Model file for the job. Use its own axes, mm. Coordinates: 2 decimals unless noted, no trailing zeros. Order: outer loops, then holes, each group sorted by start corner. A loop starts at its lowest first (then second) coordinate and runs counter-clockwise, first axis right, second up. Notation, with made-up numbers: (66.5, 88) -> (108.5, 88) arc R13 ccw to (108.5, 92) -> close; hole circle Ø11 at (84.5, 35.25). An arc over 180 degrees is marked (long way). Return JSON: item names as keys, results as strings. Group by question number.
1) Probe line 1 (Z direction, x = 9, y = -0.3); line 2 (Z direction, x = 30.5, y = -0.4); line 3 (X direction, y = -0.35, z = -22). List the from-to ranges inside material, lowest first.
2) Cut at D-D (x = 19). Write the cut outline in (y, z).
3) Cut at B-B (y = -0.05). Write the cut outline in (x, z).
4) Cut at C-C (z = -50). Write the cut outline in (x, y).
5) Flat gauge pins, fed straight in: pin 1 (3.5 mm diameter, centred on x = 9, z = 40, fed in from -Y); pin 2 (0.5 mm diameter, centred on x = 29.5, y = 0, fed in from +Z). Where does each tip first touch, or does it go through?
6) Cut at A-A (z = 77). Write the cut outline in (x, y).
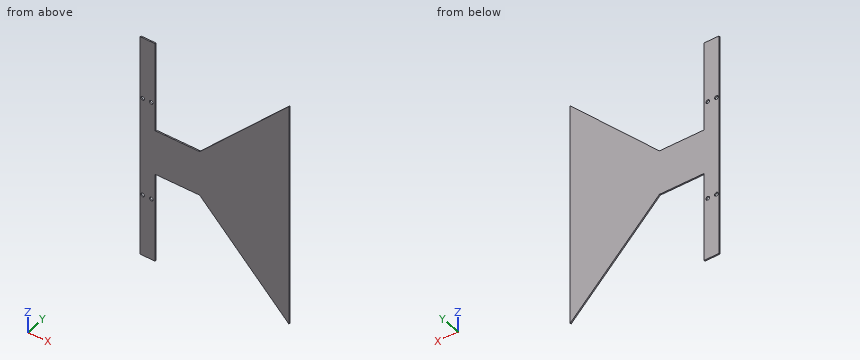
from build123d import *

# Parameters (mm, degrees)
F0_R     = 1.5
F0_W     = 36
F0_H     = 36
F1_DEPTH = 0.5


with BuildPart() as f1:
    # F0 (on Front) → F1 (new body, symmetric)
    with BuildSketch(Plane.XZ):
        Polygon((12, 90), (0, 90), (0, -90), (12, -90), (12, -18), (12, 18), align=None)
        with Locations((2, -40)):
            Circle(F0_R, mode=Mode.SUBTRACT)
        with Locations((9, -40)):
            Circle(F0_R, mode=Mode.SUBTRACT)
        with Locations((2, 40)):
            Circle(F0_R, mode=Mode.SUBTRACT)
        with Locations((9, 40)):
            Circle(F0_R, mode=Mode.SUBTRACT)
        with Locations((30, 0)):
            Rectangle(F0_W, F0_H)
        Polygon((120, 90), (48, 18), (48, -18), (120, -90), align=None)
    extrude(amount=F1_DEPTH, both=True)


solid = f1.part
Answers below:
{
 "1": {"line 1": "z = -90 to -41.5, -38.5 to 38.5, 41.5 to 90", "line 2": "z = -18 to 18", "line 3": "x = 0 to 12, 52 to 120"},
 "2": {"outline": "(-0.5, -18) -> (0.5, -18) -> (0.5, 18) -> (-0.5, 18) -> close"},
 "3": {"outline": "(0, -90) -> (12, -90) -> (12, -18) -> (48, -18) -> (120, -90) -> (120, 90) -> (48, 18) -> (12, 18) -> (12, 90) -> (0, 90) -> close; hole circle Ø3 at (2, -40); hole circle Ø3 at (2, 40); hole circle Ø3 at (9, -40); hole circle Ø3 at (9, 40)"},
 "4": {"outline": "(0, -0.5) -> (12, -0.5) -> (12, 0.5) -> (0, 0.5) -> close; (80, -0.5) -> (120, -0.5) -> (120, 0.5) -> (80, 0.5) -> close"},
 "5": {"pin 1": "stops at y = -0.5", "pin 2": "stops at z = 18"},
 "6": {"outline": "(0, -0.5) -> (12, -0.5) -> (12, 0.5) -> (0, 0.5) -> close; (107, -0.5) -> (120, -0.5) -> (120, 0.5) -> (107, 0.5) -> close"}
}
